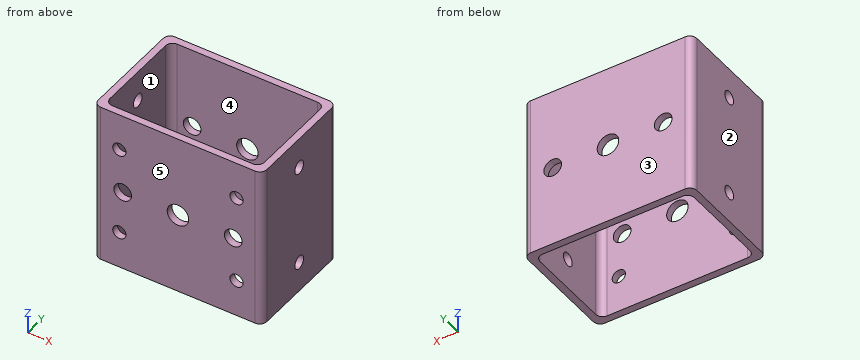
Autodesk Inventor part; units mm, degrees
ref_plane "YZ Plane" through (0, 0, 0) normal (1, 0, 0) x (0, 1, 0)
ref_plane "XZ Plane" through (0, 0, 0) normal (0, 1, 0) x (-1, 0, 0)
ref_plane "XY Plane" through (0, 0, 0) normal (0, 0, 1) x (1, 0, 0)
sketch "Sketch1" plane through (0, 0, 0) normal (0, 0, 1) x (1, 0, 0)
  line L0 (0, 0) -> (76.2, 0)
  line L1 (76.2, 0) -> (76.2, 50.8)
  line L2 (76.2, 50.8) -> (0, 50.8)
  line L3 (0, 50.8) -> (0, 0)
  dimension "d0" = 76.2
  dimension "d1" = 50.8
extrude "Extrusion1" add sketch "Sketch1" along normal blind 73.66
shell "Shell1" thickness 3.175 removed faces 2 at (50.8, 16.9333, 0) at (50.8, 16.9333, 73.66)
sketch "Sketch2" plane through (0, 0, 0) normal (0, -1, 0) x (1, 0, 0)
  line L0 (11.6, 16.83) -> (64.6, 16.83) construction
  line L1 (64.6, 16.83) -> (64.6, 56.83) construction
  line L2 (64.6, 56.83) -> (11.6, 56.83) construction
  line L3 (11.6, 56.83) -> (11.6, 16.83) construction
  circle A0 centre (11.6, 16.83) radius 3
  circle A1 centre (11.6, 56.83) radius 3
  circle A2 centre (64.6, 56.83) radius 3
  circle A3 centre (64.6, 16.83) radius 3
  line L4 (0, 0) -> (0, 73.66) construction
  line L5 (0, 0) -> (76.2, 0) construction
  point P0 (11.6, 36.83)
  point P1 (0, 36.83)
  point P2 (38.1, 16.83)
  point P3 (38.1, 0)
  dimension "d5" = 6
  dimension "d6" = 53
  dimension "d7" = 40
extrude "Extrusion2" cut sketch "Sketch2" against normal blind 23.8125
sketch "Sketch3" plane through (0, 50.8, 0) normal (0, 1, 0) x (1, 0, 0)
  line L0 (76.2, 0) -> (0, 0) construction
  line L1 (0, 0) -> (0, -73.66) construction
  circle A0 centre (13.1, -36.83) radius 4
  circle A1 centre (63.1, -36.83) radius 4
  line L2 (63.1, -36.83) -> (13.1, -36.83) construction
  circle A2 centre (38.1, -36.83) radius 4.8652
  point P0 (38.1, 0)
  point P1 (0, -36.83)
  point P2 (38.1, 0)
  dimension "d10" = 8
  dimension "d22" = 50
extrude "Extrusion3" cut sketch "Sketch3" against normal blind 101.6
fillet "Fillet1" radius 3.175 8 edges at (0, 50.8, 36.83) (76.2, 50.8, 36.83) (0, 0, 36.83) (3.175, 3.175, 36.83) (73.025, 3.175, 36.83) (3.175, 47.625, 36.83) (73.025, 47.625, 36.83) (76.2, 0, 36.83)
sketch "Sketch4" plane through (3.175, 50.8, 0) normal (0, 1, 0) x (1, 0, 0)
  circle A0 centre (8.425, -18.1) radius 4
  circle A1 centre (8.425, -58.1) radius 4
  circle A2 centre (61.425, -18.1) radius 4
  circle A3 centre (61.425, -58.1) radius 4
  circle A4 centre (8.425, -18.1) radius 3 construction
  circle A5 centre (61.425, -18.1) radius 3 construction
  circle A6 centre (8.425, -58.1) radius 3 construction
  circle A7 centre (61.425, -58.1) radius 3 construction
  point P0 (-3.175, 0)
  dimension "d14" = 8
extrude "Extrusion4" [suppressed]
sketch "Sketch5" plane through (76.2, 3.175, 0) normal (1, 0, 0) x (0, 0, -1)
  circle A0 centre (-59.83, 22.225) radius 3
  circle A1 centre (-13.83, 22.225) radius 3
  line L0 (-59.83, 22.225) -> (-13.83, 22.225) construction
  line L1 (-40.83, 47.625) -> (-32.83, 47.625) construction
  line L2 (0, 47.625) -> (-73.66, 47.625) construction
  line L3 (-73.66, 47.625) -> (0, 47.625) construction
  line L4 (0, 0) -> (0, 44.45) construction
  point P0 (0, -3.175)
  point P1 (-62.1, 47.625)
  point P2 (-54.1, 47.625)
  point P3 (-22.1, 47.625)
  point P4 (-14.1, 47.625)
  point P5 (-62.1, 47.625)
  point P6 (-54.1, 47.625)
  point P7 (-22.1, 47.625)
  point P8 (-14.1, 47.625)
  point P9 (-36.83, 47.625)
  point P10 (-36.83, 22.225)
  point P11 (0, 22.225)
  dimension "d17" = 6
  dimension "d18" = 46
extrude "Extrusion5" cut sketch "Sketch5" against normal through all
properties part number "2x3_Tube"
Model file for the job. Use its own axes, mm. Face numbers are marked on the shaded views. A direction names the side the tool comes from. Coordinates: 2 decimals unless noted, no trailing zeros. Order: outer loops, then holes, each group sorted by start corner. A loop starts at its lowest first (then second) coordinate and runs counter-clockwise, first axis right, second up. Notation, with made-up numbers: (36, 80.5) -> (74, 80.5) arc R24 ccw to (74, 91.5) -> close; hole circle Ø9 at (76, 68). An arc over 180 degrees is marked (long way). Return JSON: item names as keys, results as strings. Group by question number.
Item 1: Saw through at B-B on y = 25.4. Write the cut outline in (x, z) (3 decimals), then the cut area to 3 significant figures.
Item 2: Pull direction Y, two halves, no side cores. Call the marked faces 3, 4 and 5: pulls with the +Y half, pulls with the -Y half, needs draft (parallel to the pull), parting line crosses it, or undercut.
Item 3: Flat gauge pin, fed straight in: P1, Ø5, axis at x = 11.6, z = 16.83, coming from the -Y side (3 decimals). Where does the tip first touch, or does it go through?
Item 4: Saw through at A-A on x = 51. Write the cut outline in (y, z) (3 decimals), then the cut area to 3 significant figures.
Item 5: Saw through at D-D on y = 34. Write the cut outline in (x, z) (3 decimals).
Item 6: Saw through at C-C on x = 38.1. Write the cut outline in (y, z) (3 decimals), then the cut area to 3 significant figures.
Item 7: Wall check: line 1 along X through (y, z) = (9, 65) (3 decimals); line 2 along Y through (x, z) = (18, 5) (3 decimals); line 3 along X through (y, z) = (2.2, 36.83). Give the ranges that are in metal, low to high. Write a range as [from, to].
Item 8: Tool access for the marked faces 1 and 2: list every direction of +Z, -Z, +X, -X, +Y, -Y with a clear straight run to the whole face (end or side of a thin tool).
Values found:
{
 "1": {"outline": "(0, 0) -> (3.175, 0) -> (3.175, 10.83) -> (0, 10.83) -> close; (0, 16.83) -> (3.175, 16.83) -> (3.175, 56.83) -> (0, 56.83) -> close; (0, 62.83) -> (3.175, 62.83) -> (3.175, 73.66) -> (0, 73.66) -> close; (73.025, 0) -> (76.2, 0) -> (76.2, 10.83) -> (73.025, 10.83) -> close; (73.025, 16.83) -> (76.2, 16.83) -> (76.2, 56.83) -> (73.025, 56.83) -> close; (73.025, 62.83) -> (76.2, 62.83) -> (76.2, 73.66) -> (73.025, 73.66) -> close", "area": "392 mm2"},
 "2": {"face 3": "pulls with the +Y half", "face 4": "undercut", "face 5": "pulls with the -Y half"},
 "3": {"P1": "stops at y = 47.625"},
 "4": {"outline": "(0, 0) -> (3.175, 0) -> (3.175, 73.66) -> (0, 73.66) -> close; (47.625, 0) -> (50.8, 0) -> (50.8, 73.66) -> (47.625, 73.66) -> close", "area": "468 mm2"},
 "5": {"outline": "(0, 0) -> (3.175, 0) -> (3.175, 73.66) -> (0, 73.66) -> close; (73.025, 0) -> (76.2, 0) -> (76.2, 73.66) -> (73.025, 73.66) -> close"},
 "6": {"outline": "(0, 0) -> (3.175, 0) -> (3.175, 31.965) -> (0, 31.965) -> close; (0, 41.695) -> (3.175, 41.695) -> (3.175, 73.66) -> (0, 73.66) -> close; (47.625, 0) -> (50.8, 0) -> (50.8, 31.965) -> (47.625, 31.965) -> close; (47.625, 41.695) -> (50.8, 41.695) -> (50.8, 73.66) -> (47.625, 73.66) -> close", "area": "406 mm2"},
 "7": {"line 1": "x = [0, 3.175], [73.025, 76.2]", "line 2": "y = [0, 3.175], [47.625, 50.8]", "line 3": "x = [0.15, 9.1], [17.1, 33.23], [42.97, 59.1], [67.1, 76.05]"},
 "8": {"face 1": "+Z, -Z", "face 2": "+Z, -Z, -X, +Y, -Y"}
}
